Geometry check sheet. Reference: drawing and pictorial views, mm from the part's lowest x, y, z. Round coordinates to 2 decimals unless told otherwise and drop trailing zeros. Loops run counter-clockwise (first coordinate to the right, second up) from the corner with the lowest first, then second, coordinate; pieces in that order, holes last. Notation, with made-up numbers: (44, 68.25) - (57, 68.25) arc R11 ccw to (57, 86.25) - close; hole circle Ø3 at (-2.75, -29.5). An arc over 180 degrees is marked (long way). Return JSON: item names as keys, results as strings.
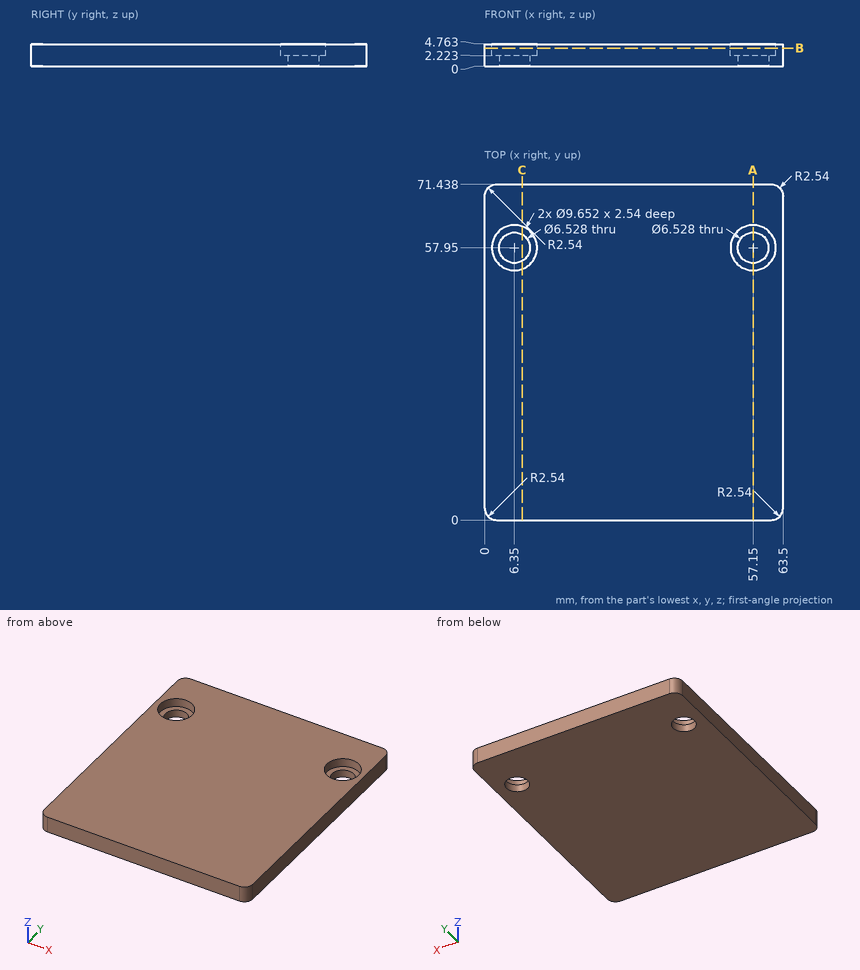
Q1. Depth check by flat-ended pin: P1, Ø5, axis at x = 6.5, y = 60, coming from the +Z side; P2, Ø2, axis at x = 46.5, z = 3.5, coming from the -Y side. Enter the tip coordinate at first touch or a pass-through.
Answer key:
{"P1": "stops at z = 2.22", "P2": "stops at y = 0"}
Q2. Scan lines: probe 1 along X at (y, z) = (60, 2.9); probe 2 along Y at (x, z) = (57.15, 3.7) (1 decimal); probe 3 along Y at (x, z) = (6.35, 1.5) (1 decimal). Record each from-to range of solid material in increasing order. Write a range as [from, to].
Answer key:
{"probe 1": "x = [0, 1.98], [10.72, 52.78], [61.52, 63.5]", "probe 2": "y = [0, 53.1], [62.8, 71.4]", "probe 3": "y = [0, 54.7], [61.2, 71.4]"}
Q3. Sectioned sample at B-B (z = 3.9). State how many separate pieces and enclosed holes the cut face has, plus the area to 3 significant figures.
Answer key:
{"separate pieces": "1", "enclosed holes": "2", "area": "4,380 mm²"}
Q4. Sectioned sample at C-C (x = 8). Enter the section's corners in (y, z) (1 decimal).
Answer key:
{"outline": "(0, 0) - (55.1, 0) - (55.1, 2.2) - (53.4, 2.2) - (53.4, 4.8) - (0, 4.8) - close; (60.8, 0) - (71.4, 0) - (71.4, 4.8) - (62.5, 4.8) - (62.5, 2.2) - (60.8, 2.2) - close"}
Q5. Sectioned sample at A-A (x = 57.15). Enter the section's corners in (y, z) (1 decimal), plus the area to 3 significant figures.
Answer key:
{"outline": "(0, 0) - (54.7, 0) - (54.7, 2.2) - (53.1, 2.2) - (53.1, 4.8) - (0, 4.8) - close; (61.2, 0) - (71.4, 0) - (71.4, 4.8) - (62.8, 4.8) - (62.8, 2.2) - (61.2, 2.2) - close", "area": "301 mm²"}
